from build123d import *

# Parameters (mm, degrees)
BOSS_EXTRUDE1_DEPTH = 6.35
BOSS_EXTRUDE2_START = -3.81
SKETCH2_R           = 3.175
SKETCH2_R_2         = 1.27
BOSS_EXTRUDE2_DEPTH = 16.51


with BuildPart() as part:
    # Sketch1 → Boss-Extrude1 (new body)
    with BuildSketch(Plane(origin=(0, 0, 0), x_dir=(1, 0, 0), z_dir=(0, 1, 0))):
        Polygon((-25.881030621, 0), (-23.020766125, 23.020766125), (0, 0), align=None)
    extrude(amount=BOSS_EXTRUDE1_DEPTH)

    # Sketch2 → Boss-Extrude2 (add)
    with BuildSketch(Plane(origin=(0, 0, 0), x_dir=(0, 0, -1), z_dir=(1, 0, 0)).offset(BOSS_EXTRUDE2_START)):
        with Locations((-3.175, 3.175)):
            Circle(SKETCH2_R)
        with Locations((-3.175, 3.175)):
            Circle(SKETCH2_R_2, mode=Mode.SUBTRACT)
        with BuildLine():
            ThreePointArc((-3.174999994, 6.35), (-0.929935968, 5.420064028), (0, 3.175))
            Line((0, 3.175), (0, 6.35))
            Line((0, 6.35), (-3.174999994, 6.35))
        make_face()
        with BuildLine():
            ThreePointArc((0, 3.175), (-0.92993597, 0.92993597), (-3.175, 0))
            Line((-3.175, 0), (0, 0))
            Line((0, 0), (0, 3.175))
        make_face()
        with BuildLine():
            Line((-6.35, 3.175), (-6.35, 0))
            Line((-6.35, 0), (-3.175, 0))
            ThreePointArc((-3.175, 0), (-5.42006403, 0.92993597), (-6.35, 3.175))
        make_face()
    extrude(amount=-BOSS_EXTRUDE2_DEPTH)


solid = part.part
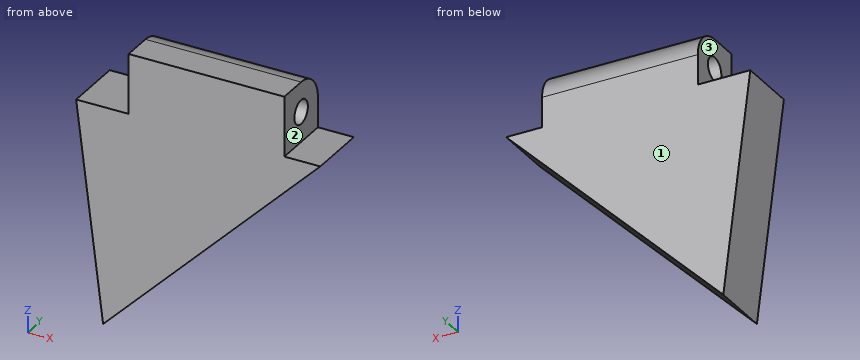
Geometry: final body of the model. Coordinates: model frame, mm. Face numbers are marked on the shaded views. A direction names the side the tool comes from. Give positions to 0.01 mm unless a question says otherwise; leave off trailing zeros. Write each loop counter-clockwise with the first axis right and the second up, starting at its lowest first coordinate (ties: lowest second). Pieces come first, ordered by that corner, then holes. Notation, with made-up numbers: (61, 13.25) -> (108, 13.25) arc R27 cw to (108, 52.25) -> close; hole circle Ø9 at (21, 19.5). An arc over 180 degrees is marked (long way). Answer as a JSON object with one key per item and string values.
1. Contact query for flat-ended pins moving along their axis: pin 1 (1.5 mm diameter, centred on y = 2, z = -10, fed in from -X); pin 2 (1.5 mm diameter, centred on x = -15, y = 2.5, fed in from -Z); pin 3 (1 mm diameter, centred on y = 4.5, z = -2.5, fed in from -X). Output: stop coordinate, or through.
Ans:
{"pin 1": "stops at x = -24.73", "pin 2": "stops at z = -15.75", "pin 3": "stops at x = -25.63"}
2. Cut plane C-C on y = 5. Output: boundary loops of the cut face in (x, z).
Ans:
{"outline": "(-25.88, 0) -> (-23.02, -23.02) -> (0, 0) -> (-3.81, 0) -> (-3.81, 5.77) -> (-20.32, 5.77) -> (-20.32, 0) -> close"}
3. Cut plane B-B on x = -7. Output: boundary loops of the cut face in (y, z) (3 decimals), and give its area (3 significant figures).
Ans:
{"outline": "(0, -7) -> (6.35, -7) -> (6.35, 3.175) arc R3.175 ccw to (3.175, 6.35) -> (0, 6.35) -> close; hole circle Ø2.54 at (3.175, 3.175)", "area": "77.5 mm^2"}
4. Cut plane A-A on y = 2.5. Output: boundary loops of the cut face in (x, z).
Ans:
{"outline": "(-25.88, 0) -> (-23.02, -23.02) -> (0, 0) -> (-3.81, 0) -> (-3.81, 2.1) -> (-20.32, 2.1) -> (-20.32, 0) -> close; (-20.32, 4.25) -> (-3.81, 4.25) -> (-3.81, 6.35) -> (-20.32, 6.35) -> close"}
5. Cut plane D-D on x = -1.75. Output: boundary loops of the cut face in (y, z).
Ans:
{"outline": "(0, -1.75) -> (6.35, -1.75) -> (6.35, 0) -> (0, 0) -> close"}
6. Access query for the marked faces 1, 2 and 3. Directions: +Z, -Z, +X, -X, +Y, -Y. A direction counts if a zero-diameter tool reaches every point of the face in a straight line with its end or side. Return the directions, or none.
Ans:
{"face 1": "+Z, -Z, +X, -X, +Y", "face 2": "+Z, +X, +Y, -Y", "face 3": "+Z, -X, +Y, -Y"}
7. Ray query, probe 1 along X at (y, z) = (3.5, 0.75); probe 2 along Z at (x, y) = (-5.75, 4); probe 3 along Z at (x, y) = (-16.25, 3.75). Return the intervals inside material, ascending. Write a range as from..to.
Ans:
{"probe 1": "x = -20.32..-3.81", "probe 2": "z = -5.75..2.21, 4.14..6.24", "probe 3": "z = -16.25..2.04, 4.31..6.3"}
